Geometry check sheet. Reference: the model listing, model coordinates, mm. A direction names the side the tool comes from. Give positions to 0.01 mm unless a question says otherwise; leave off trailing zeros. Loops run counter-clockwise (first coordinate to the right, second up) from the corner with the lowest first, then second, coordinate; pieces in that order, holes last. Notation, with made-up numbers: (-5, 7) - (50, 7) arc R28 ccw to (50, 35) - close; hole circle Ø6 at (35.25, -25). An arc over 180 degrees is marked (long way). Use a Markdown table: item, result. Add a question column.
1. Cross-section at B-B on y = 1.75. Enter the section's corners in (x, z), and give its area (3 significant figures).
2. Cross-section at C-C on z = 8. Enter the section's corners in (x, y) (3 decimals).
3. Draft check along Y on faces 1 (the flat face through (-10, 13, 16.51)), 2 (the flat face through (0, 22.225, 14)), 3 (the cylindrical face through (-1.816, 19.359, -14.208)). Enter one of: pulls with the +Y half, pulls with the -Y half, needs draft (parallel to the pull), parting line crosses it, or undercut.
4. Cross-section at A-A on x = 5.5. Enter the section's corners in (y, z) (3 decimals), and give its area (3 significant figures).
5. Material ranges on L1, parallel to X at y = 2.25, z = 0; L2, parallel to Z at x = 16, y = 14.25; L3, parallel to X at y = 1, z = -16.51, recorded low to high.
6. Set-up check for faces 4 (the flat face through (-16.51, 13, 0)), 5 (the flat face through (16.51, 13, -10)), 6 (the flat face through (-10, 13, -16.51)), 7 (the flat face through (12.7, 11, 0)), 8 (the flat face through (10, 13, 16.51)): record each of +Z, -Z, +X, -X, +Y, -Y from which the full face is reachable in a straight line by a thin tool's end or side.
7. Depth check by flat-ended pin: P1, Ø4, axis at x = 16.51, z = 0, coming from the -Y side; P2, Ø3, axis at x = 15, y = 16, coming from the -Z side; P3, Ø4, axis at x = 0, y = 16.51, coming from the -Z side; P4, Ø12, axis at y = 10, z = 6, coming from the -X side. Enter the tip coordinate at first touch or a pass-through.
8. Cross-section at D-D on x = 0. Count the separate pieces of the cut face and the enclosed holes in it, and give its area (3 significant figures).
from build123d import *

# Parameters (mm, degrees)
SKETCH1_W           = 38.1
SKETCH1_H           = 38.1
BOSS_EXTRUDE1_DEPTH = 3.175
SKETCH2_W           = 33.02
SKETCH2_H           = 33.02
BOSS_EXTRUDE2_DEPTH = 19.05
SKETCH3_W           = 25.4
SKETCH3_H           = 25.4
CUT_EXTRUDE1_DEPTH  = 23.225
SKETCH4_R           = 1.6002
CUT_EXTRUDE2_DEPTH  = 4.175
CIRPATTERN1_COUNT   = 4
SKETCH6_R           = 3.3782
CUT_EXTRUDE4_DEPTH  = 36.56
SKETCH10_R          = 3.175
CIRPATTERN3_COUNT   = 4


with BuildPart() as part:
    # Sketch1 → Boss-Extrude1 (new body)
    with BuildSketch(Plane(origin=(0, 0, 0), x_dir=(1, 0, 0), z_dir=(0, 1, 0))):
        Rectangle(SKETCH1_W, SKETCH1_H)
    extrude(amount=BOSS_EXTRUDE1_DEPTH)

    # Sketch2 → Boss-Extrude2 (add)
    with BuildSketch(Plane(origin=(0, 3.175, 0), x_dir=(1, 0, 0), z_dir=(0, 1, 0))):
        Rectangle(SKETCH2_W, SKETCH2_H)
    extrude(amount=BOSS_EXTRUDE2_DEPTH)

    # Sketch3 → Cut-Extrude1 (cut, through all)
    with BuildSketch(Plane(origin=(0, 22.225, 0), x_dir=(1, 0, 0), z_dir=(0, 1, 0))):
        Rectangle(SKETCH3_W, SKETCH3_H)
    extrude(amount=-CUT_EXTRUDE1_DEPTH, mode=Mode.SUBTRACT)

    # Sketch4 → Cut-Extrude2 (cut, through all)
    with BuildSketch(Plane(origin=(0, 3.175, 0), x_dir=(1, 0, 0), z_dir=(0, 1, 0))):
        with Locations((16.51, 0)):
            Circle(SKETCH4_R)
    cut_extrude2 = extrude(amount=-CUT_EXTRUDE2_DEPTH, mode=Mode.SUBTRACT)

    # CirPattern1: Cut-Extrude2 ×4 about axis, 1 skipped
    cirpattern1_axis = Axis((0, 0, 0), (0, 1, 0))
    add([cut_extrude2.rotate(cirpattern1_axis, i * 360 / CIRPATTERN1_COUNT) for i in range(1, CIRPATTERN1_COUNT) if i not in (2,)], mode=Mode.SUBTRACT)

    # Sketch6 → Cut-Extrude4 (cut, through all)
    with BuildSketch(Plane(origin=(0, 0, -16.51), x_dir=(-1, 0, 0), z_dir=(0, 0, -1))):
        with Locations((0, 16.51)):
            Circle(SKETCH6_R)
    extrude(amount=-CUT_EXTRUDE4_DEPTH, mode=Mode.SUBTRACT)

    # Cut-Sweep2: sweep along a path in Sketch9
    with BuildLine(Plane.XY) as cut_sweep2_path:
        Line((16.51, 3.175), (17.78, 22.225))
    # Sketch10 → Cut-Sweep2 (sweep, cut)
    with BuildSketch(Plane(origin=(0, 3.175, 0), x_dir=(1, 0, 0), z_dir=(0, 1, 0))):
        with Locations((16.51, 0)):
            Circle(SKETCH10_R)
    cut_sweep2 = sweep(path=cut_sweep2_path.line, mode=Mode.SUBTRACT)

    # CirPattern3: Cut-Sweep2 ×4 about axis, 1 skipped
    cirpattern3_axis = Axis((0, -1.42875, 0), (0, 1, 0))
    add([cut_sweep2.rotate(cirpattern3_axis, i * 360 / CIRPATTERN3_COUNT) for i in range(1, CIRPATTERN3_COUNT) if i not in (2,)], mode=Mode.SUBTRACT)


solid = part.part
Values found:
| question | item | result |
|---|---|---|
| 1 | outline | (-19.05, -19.05) - (19.05, -19.05) - (19.05, 19.05) - (-19.05, 19.05) - close; hole (-12.7, -12.7) - (12.7, -12.7) - (12.7, 12.7) - (-12.7, 12.7) - close; hole circle Ø3.2 at (0, -16.51); hole circle Ø3.2 at (0, 16.51); hole circle Ø3.2 at (16.51, 0) |
| 1 | area | 782 mm2 |
| 2 | outline | (-19.05, 0) - (-12.7, 0) - (-12.7, 22.225) - (-16.51, 22.225) - (-16.51, 3.175) - (-19.05, 3.175) - close; (12.7, 0) - (19.05, 0) - (19.05, 3.175) - (16.51, 3.175) - (16.51, 22.225) - (12.7, 22.225) - close |
| 3 | face 1 | needs draft |
| 3 | face 2 | pulls with the +Y half |
| 3 | face 3 | undercut |
| 4 | outline | (0, -19.05) - (3.175, -19.05) - (3.175, -16.51) - (22.225, -16.51) - (22.225, -12.7) - (0, -12.7) - close; (0, 12.7) - (22.225, 12.7) - (22.225, 16.51) - (3.175, 16.51) - (3.175, 19.05) - (0, 19.05) - close |
| 4 | area | 185 mm2 |
| 5 | L1 | x = -19.05 to -12.7, 12.7 to 14.91, 18.11 to 19.05 |
| 5 | L2 | z = -16.51 to -2.92, 2.92 to 16.51 |
| 5 | L3 | x = -19.05 to -1.6, 1.6 to 19.05 |
| 6 | face 4 | +Z, -Z, -X, +Y |
| 6 | face 5 | +Z, -Z, +X, +Y |
| 6 | face 6 | -Z, +X, -X, +Y |
| 6 | face 7 | +Y, -Y |
| 6 | face 8 | +Z, +X, -X, +Y |
| 7 | P1 | stops at y = 0 |
| 7 | P2 | stops at z = -16.51 |
| 7 | P3 | passes through |
| 7 | P4 | stops at x = -16.51 |
| 8 | separate pieces | 6 |
| 8 | enclosed holes | 0 |
| 8 | area | 47.8 mm2 |
